Geometry: final body of the model. Coordinates: model frame, mm. Face numbers are marked on the shaded views. A direction names the side the tool comes from. Give positions to 0.01 mm unless a question says otherwise; leave off trailing zeros. Order: outer loops, then holes, each group sorted by start corner. A loop starts at its lowest first (then second) coordinate and runs counter-clockwise, first axis right, second up. Notation, with made-up numbers: (80.5, -16) -> (138.5, -16) arc R3 ccw to (138.5, -12) -> close; hole circle Ø4 at (-0.5, -6). An arc over 180 degrees is marked (long way). One line per item, written item: value. Start each with the question number.
```python
from build123d import *

# Parameters (mm, degrees)
SKETCH1_R           = 8
BOSS_EXTRUDE1_DEPTH = 12.8
SKETCH3_R           = 7.65
BOSS_EXTRUDE3_DEPTH = 27
CUT_EXTRUDE1_DEPTH  = 27
BOSS_EXTRUDE4_DEPTH = 25.4
SKETCH8_W           = 1.2
SKETCH8_H           = 2
BOSS_EXTRUDE5_DEPTH = 5


with BuildPart() as part:
    # Sketch1 → Boss-Extrude1 (new body)
    with BuildSketch(Plane.XY):
        Circle(SKETCH1_R)
    extrude(amount=BOSS_EXTRUDE1_DEPTH)

    # Sketch3 → Boss-Extrude3 (add)
    with BuildSketch(Plane(origin=(0, 0, 0), x_dir=(-1, 0, 0), z_dir=(0, 0, -1))):
        Circle(SKETCH3_R)
    extrude(amount=BOSS_EXTRUDE3_DEPTH)

    # Sketch4 → Cut-Extrude1 (cut)
    with BuildSketch(Plane(origin=(0, 0, -27), x_dir=(-1, 0, 0), z_dir=(0, 0, -1))):
        with BuildLine():
            Line((-4.745787606, -6), (4.745787606, -6))
            ThreePointArc((4.745787606, -6), (0, -7.65), (-4.745787606, -6))
        make_face()
        with BuildLine():
            Line((-4.745787606, 6), (4.745787606, 6))
            ThreePointArc((4.745787606, 6), (0, 7.65), (-4.745787606, 6))
        make_face()
    extrude(amount=-CUT_EXTRUDE1_DEPTH, mode=Mode.SUBTRACT)

    # Sketch7 → Boss-Extrude4 (add)
    with BuildSketch(Plane.XY.offset(12.8)):
        with BuildLine():
            Line((-1.160818677, 0.95), (1.160818677, 0.95))
            ThreePointArc((1.160818677, 0.95), (0, -1.5), (-1.160818677, 0.95))
        make_face()
    extrude(amount=BOSS_EXTRUDE4_DEPTH)

    # Sketch8 → Boss-Extrude5 (add)
    with BuildSketch(Plane(origin=(0, 0, -27), x_dir=(-1, 0, 0), z_dir=(0, 0, -1))):
        with Locations((-5.5, 0)):
            Rectangle(SKETCH8_W, SKETCH8_H)
        with Locations((5.5, 0)):
            Rectangle(SKETCH8_W, SKETCH8_H)
    extrude(amount=BOSS_EXTRUDE5_DEPTH)


solid = part.part
```
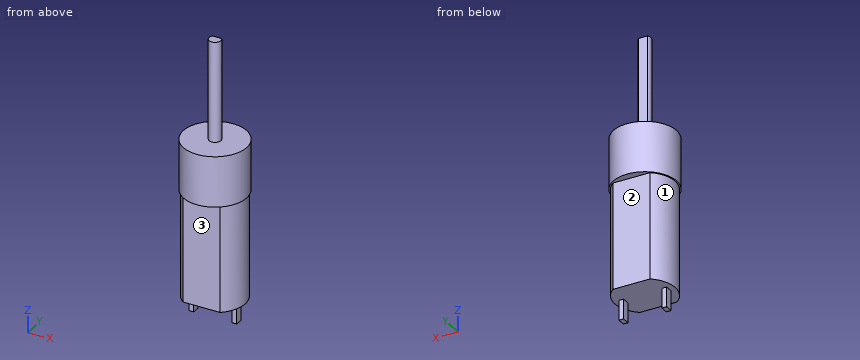
1. Cut plane A-A, the plane x = 0. Return loops of the section in (y, z), then the cut area to 3 significant figures.
2. Cut plane D-D, the plane z = 11.5. Return loops of the section in (x, y).
3. Cut plane C-C, the plane z = 34. Return loops of the section in (x, y).
4. Cut plane B-B, the plane y = 0. Return loops of the section in (x, z), then the cut area to 3 significant figures.
5. Access query for the marked faces 1, 2 and 3. Directions: +Z, -Z, +X, -X, +Y, -Y. A direction counts if a zero-diameter tool reaches every point of the face in a straight line with its end or side. Return the directions, or none.
6. Material intervals for L1, parallel to X at y = -0.25, z = -27.5; L2, parallel to Z at x = 0, y = 5.25; L3, parallel to Y at x = 5, z = -29, sorted ascending. Write a range as [from, to].
7. Pin query (flat end, axial travel): P1, Ø1, axis at y = 5.5, z = -22, coming from the +X side; P2, Ø1.2, axis at x = -0.5, z = 21.5, coming from the +Y side; P3, Ø1, axis at x = 5.5, z = -29, coming from the -Y side; P4, Ø1, axis at y = 3, z = 23.5, coming from the -X side. Return the tip coordinate at first contact, or that it passes through.
Answers follow:
1. outline: (-8, 0) -> (-6, 0) -> (-6, -27) -> (6, -27) -> (6, 0) -> (8, 0) -> (8, 12.8) -> (0.95, 12.8) -> (0.95, 38.2) -> (-1.5, 38.2) -> (-1.5, 12.8) -> (-8, 12.8) -> close
1. area: 591 mm²
2. outline: circle Ø16 at (0, 0)
3. outline: (-1.16, 0.95) arc R1.5 ccw (long way) to (1.16, 0.95) -> close
4. outline: (-8, 0) -> (-7.65, 0) -> (-7.65, -27) -> (-6.1, -27) -> (-6.1, -32) -> (-4.9, -32) -> (-4.9, -27) -> (4.9, -27) -> (4.9, -32) -> (6.1, -32) -> (6.1, -27) -> (7.65, -27) -> (7.65, 0) -> (8, 0) -> (8, 12.8) -> (1.5, 12.8) -> (1.5, 38.2) -> (-1.5, 38.2) -> (-1.5, 12.8) -> (-8, 12.8) -> close
4. area: 706 mm²
5. face 1: -Z, -X
5. face 2: -Z, +X, -X, +Y
5. face 3: -Z, +X, -X, -Y
6. L1: x = [-6.1, -4.9], [4.9, 6.1]
6. L2: z = [-27, 12.8]
6. L3: y = [-1, 1]
7. P1: stops at x = 5.79
7. P2: stops at y = 0.95
7. P3: stops at y = -1
7. P4: passes through
